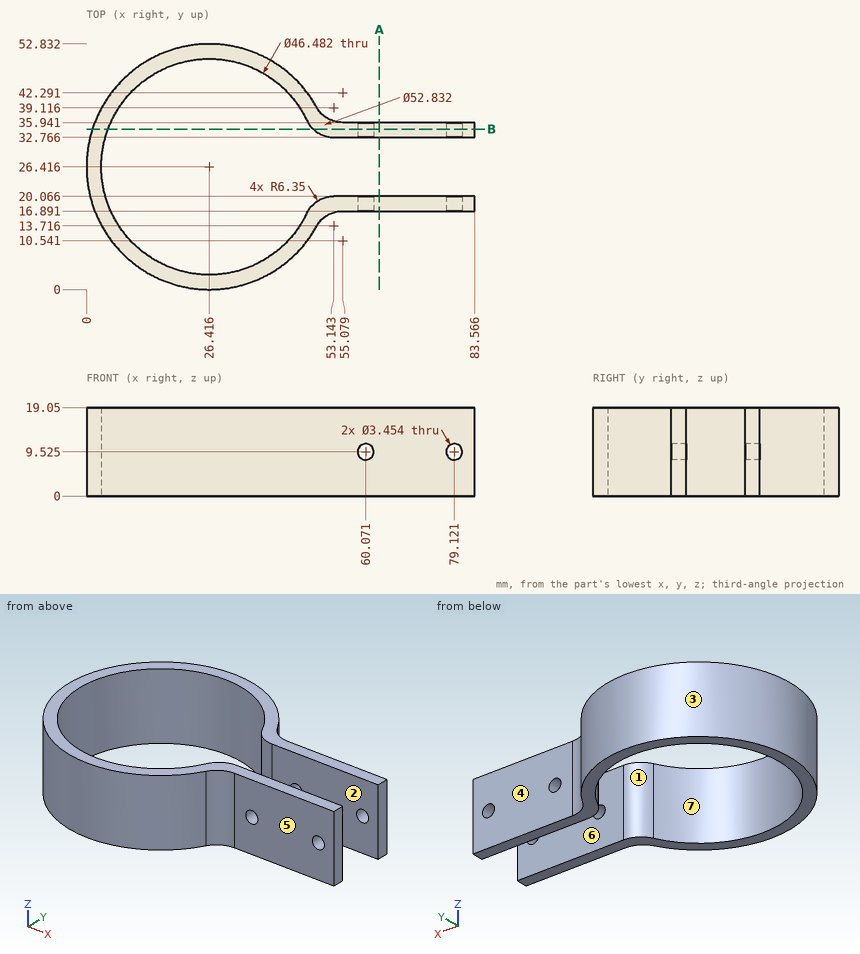
Geometry check sheet. Reference: drawing and pictorial views, mm from the part's lowest x, y, z. A direction names the side the tool comes from. Coordinates: 2 decimals unless noted, no trailing zeros. Order: outer loops, then holes, each group sorted by start corner. A loop starts at its lowest first (then second) coordinate and runs counter-clockwise, first axis right, second up.
Item 1: Mould release check, pull along X, two halves, no side actions. Record for the marked faces 1, 2 and 3: released by +X, released by -X, zero draft, split by the parting line, or undercut.
Item 2: Section check B-B (y = 34.5). Count the separate pieces of the cut face and the enclosed holes in it, plus the area to 3 significant figures.
Item 3: Depth check by flat-ended pin: pin 1 (4 mm diameter, centred on x = 79.121, z = 9.525, fed in from +Y); pin 2 (3 mm diameter, centred on y = 13, z = 8, fed in from -X); pin 3 (6 mm diameter, centred on x = 65.5, y = 28.5, fed in from +Z); pin 4 (8 mm diameter, centred on x = 33, z = 15, fed in from +Y) (1 decimal). Enter the tip coordinate at first touch or a pass-through.
Item 4: Scan lines: line 1 along Y through (x, z) = (62, 5.75); line 2 along Y through (x, z) = (30, 3.5) (1 decimal); line 3 along X through (y, z) = (40, 6.5) (1 decimal). Record each from-to range of solid material in increasing order.
Item 5: Section check A-A (x = 63). Enter the section's corners in (y, z).
Item 6: Tool access check on the marked faces 4, 5, 6 and 7. Record the directions out of +Z, -Z, +X, -X, +Y, -Y that give a thin tool (end or side, any length) a straight path to the whole face; none if there is none.
Check sheet entries:
1. face 1: undercut
1. face 2: zero draft
1. face 3: split by the parting line
2. separate pieces: 2
2. enclosed holes: 2
2. area: 708 mm2
3. pin 1: stops at y = 35.94
3. pin 2: stops at x = 2.84
3. pin 3: passes through
3. pin 4: stops at y = 52.7
4. line 1: y = 16.89 to 20.07, 32.77 to 35.94
4. line 2: y = 0.2 to 3.5, 49.4 to 52.6
4. line 3: x = 3.8 to 7.6, 45.3 to 49.1
5. outline: (16.89, 0) - (20.07, 0) - (20.07, 19.05) - (16.89, 19.05) - close; (32.77, 0) - (35.94, 0) - (35.94, 19.05) - (32.77, 19.05) - close
6. face 4: +Z, -Z, +X, +Y
6. face 5: +Z, -Z, +X, -Y
6. face 6: +Z, -Z, +X
6. face 7: +Z, -Z
